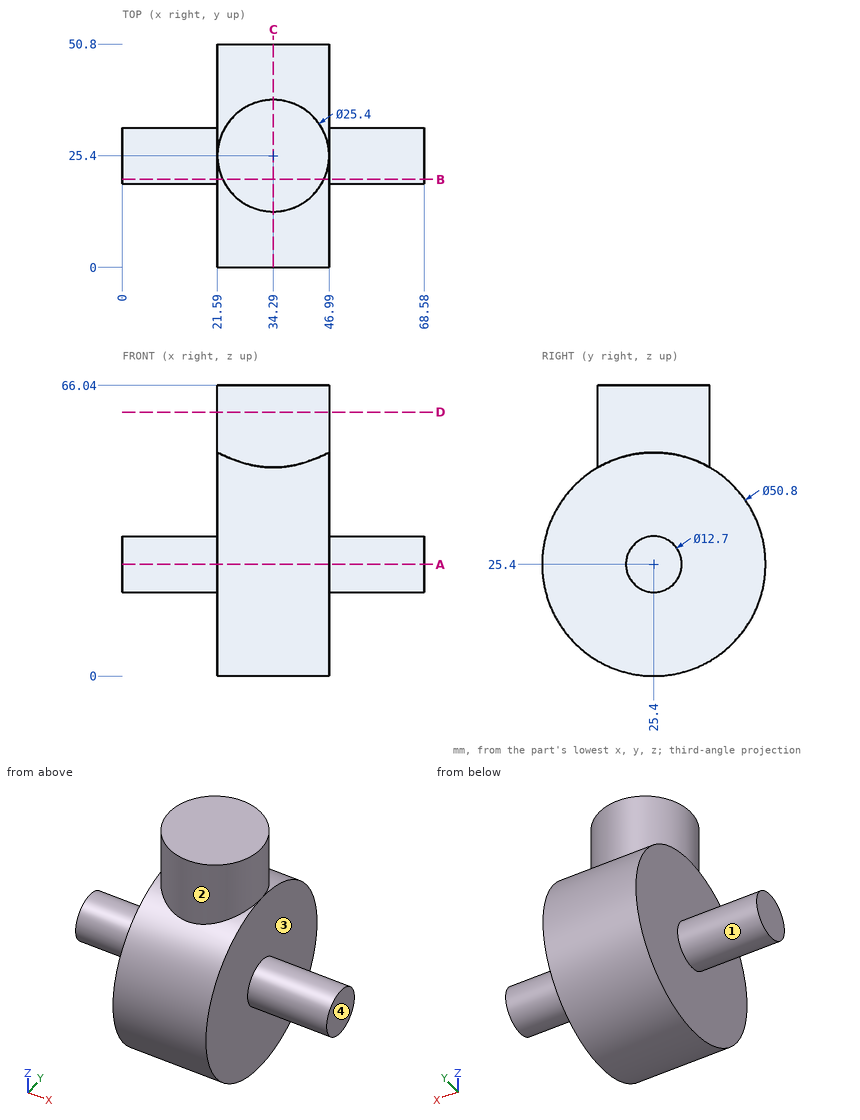
Can you work these out from the drawing? Everything is in mm from the part's minimum corner. A direction names the side the tool comes from. Give positions to 0.01 mm unless a question says otherwise; leave off trailing zeros. Write each loop counter-clockwise with the first axis right and the second up, starting at its lowest first coordinate (ties: lowest second). Pieces come first, ordered by that corner, then holes. Notation, with made-up numbers: M 61.25,87.5 L 70.25,87.5 A28 cw 70.25,115.5 Z; hole C 78,-38.75 d11. An arc over 180 degrees is marked long. Answer in a Markdown table with one row per item. Add a question column.
Item 1: Please list where these lines run through material, in increasing order: L1, parallel to X at y = 20, z = 15; L2, parallel to X at y = 33, z = 59; L3, parallel to Z at x = 61, y = 21.
Item 2: Imagine slicing it at D-D, the plane z = 60. Write out the boundary of the cut face in (x, y), plus the area to 3 significant figures.
Item 3: On a 3-axis mill with a long thin cutter (end or side, diameter ignored), from which of +Z, -Z, +X, -X, +Y, -Y can I reach the whole of each face in a straight line? I mean the marked faces 1, 2, 3 and 4. Say none if no direction works.
Item 4: Imagine slicing it at C-C, the plane x = 34.29. Write out the boundary of the cut face in (y, z), plus the area to 3 significant figures.
Item 5: Imagine slicing it at A-A, the plane z = 25.4. Write out the boundary of the cut face in (x, y).
Item 6: For pin 1 Ø4 at (x, y) = (22.5, 42) entering from -Z; pin 2 Ø8 at (y, z) = (18.5, 45) entering from +X; pin 3 Ø2 at (x, z) = (49, 23.5) entering from -Y, each with a flat end and sliding along its axis, tell me the tip position at first contact or that it passes through.
Item 7: Imagine slicing it at B-B, the plane y = 20. Write out the boundary of the cut face in (x, z).
Evaluation:
| question | item | result |
|---|---|---|
| 1 | L1 | x = 21.59 to 46.99 |
| 1 | L2 | x = 24.12 to 44.46 |
| 1 | L3 | z = 20.82 to 29.98 |
| 2 | outline | C 34.29,25.4 d25.4 |
| 2 | area | 507 mm² |
| 3 | face 1 | -X |
| 3 | face 2 | +Z |
| 3 | face 3 | +X |
| 3 | face 4 | +Z, -Z, +X, +Y, -Y |
| 4 | outline | M 12.7,47.4 A25.4 ccw long 38.1,47.4 L 38.1,66.04 L 12.7,66.04 Z |
| 4 | area | 2,440 mm² |
| 5 | outline | M 0,19.05 L 21.59,19.05 L 21.59,0 L 46.99,0 L 46.99,19.05 L 68.58,19.05 L 68.58,31.75 L 46.99,31.75 L 46.99,50.8 L 21.59,50.8 L 21.59,31.75 L 0,31.75 Z |
| 6 | pin 1 | stops at z = 4.62 |
| 6 | pin 2 | stops at x = 46.99 |
| 6 | pin 3 | stops at y = 19.11 |
| 7 | outline | M 0,22.06 L 21.59,22.06 L 21.59,0.58 L 46.99,0.58 L 46.99,22.06 L 68.58,22.06 L 68.58,28.74 L 46.99,28.74 L 46.99,50.22 L 45.78,50.22 L 45.78,66.04 L 22.8,66.04 L 22.8,50.22 L 21.59,50.22 L 21.59,28.74 L 0,28.74 Z |
